Here's how the part is built. I have some questions about the finished solid (model axes, mm). A direction names the side the tool comes from. Coordinates: 2 decimals unless noted, no trailing zeros. Write each loop counter-clockwise with the first axis right and the second up, starting at its lowest first coordinate (ties: lowest second). Pieces come first, ordered by that corner, then holes. Notation, with made-up numbers: (61.5, -33.75) -> (73.5, -33.75) arc R12 cw to (73.5, -27.75) -> close; hole circle Ø4 at (15, 54). An arc over 180 degrees is marked (long way). Answer in a Markdown table with one row per item. Add a question column.
Autodesk Inventor part; units mm, degrees
ref_plane "YZ Plane" through (0, 0, 0) normal (1, 0, 0) x (0, 1, 0)
ref_plane "XZ Plane" through (0, 0, 0) normal (0, 1, 0) x (-1, 0, 0)
ref_plane "XY Plane" through (0, 0, 0) normal (0, 0, 1) x (1, 0, 0)
sketch "Szkic2" plane through (0, 0, 0) normal (0, 1, 0) x (-1, 0, 0)
  line L0 (47.5, 5) -> (-47.5, 5)
  line L1 (-47.5, 5) -> (-47.5, -5)
  line L2 (-47.5, -5) -> (47.5, -5)
  line L3 (47.5, -5) -> (47.5, 5)
  line L4 (47.5, 5) -> (-47.5, -5) construction
  line L5 (-47.5, 5) -> (47.5, -5) construction
  line L6 (0, 24) -> (0, -27)
  point P0 (0, 0)
  dimension "d10" = 10
  dimension "d11" = 95
extrude "Wyciągnięcie proste2" add sketch "Szkic2" along normal blind 1.6
sketch "Szkic3" plane through (0, 1.6, 0) normal (0, 1, 0) x (1, 0, 0)
  line L0 (-47.5, -5) -> (47.5, -5)
  line L1 (47.5, -5) -> (47.5, 5)
  line L2 (47.5, 5) -> (-47.5, 5)
  line L3 (-47.5, 5) -> (-47.5, -5)
  line L4 (52, -8.65) -> (49.4, -5.35) construction
  line L5 (59.75, -18.7) -> (57.1, -15.35) construction
  line L6 (41.3, -1.65) -> (38.65, 1.7) construction
  line L7 (58.425, -17.025) -> (50.7, -7) construction
  line L8 (39.975, 0.025) -> (50.7, -7) construction
  line L9 (58.425, -17.025) -> (58.425, -30) construction
  line L10 (38.5214, -5) -> (47.2545, -10.7203)
  line L11 (47.2545, -10.7203) -> (53.425, -18.728)
  line L12 (53.425, -18.728) -> (53.425, -27.025)
  line L13 (41.5049, 5) -> (54.1455, -3.2797)
  line L14 (54.1455, -3.2797) -> (63.425, -15.322)
  line L15 (63.425, -15.322) -> (63.425, -27.025)
  line L16 (63.425, -27.025) -> (53.425, -27.025)
  line L17 (0, -5) -> (0, 20.232)
  line L18 (-38.5214, -5) -> (-47.2545, -10.7203)
  line L19 (-47.2545, -10.7203) -> (-53.425, -18.728)
  line L20 (-53.425, -18.728) -> (-53.425, -27.025)
  line L21 (-41.5049, 5) -> (-54.1455, -3.2797)
  line L22 (-54.1455, -3.2797) -> (-63.425, -15.322)
  line L23 (-63.425, -15.322) -> (-63.425, -27.025)
  line L24 (-63.425, -27.025) -> (-53.425, -27.025)
  point P0 (0, 0)
  point P1 (-47.5, 1.0732)
  point P2 (47.5, 1.0732)
  dimension "d17" = 5
  dimension "d18" = 5
  dimension "d19" = 10
extrude "Wyciągnięcie proste3" add sketch "Szkic3" against normal up to surface (1.6 mm away) contours L0 L18 L19 L20 L24 L23 L22 L21 L3 | L0 L1 L13 L14 L15 L16 L12 L11 L10
extrude "Wyciągnięcie proste4" cut sketch "Szkic3" against normal through all contours L3 L2 L21 | L2 L1 L13
sketch "Szkic4" plane through (0, 1.6, 0) normal (0, 1, 0) x (1, 0, 0)
  line L0 (-41.5049, 5) -> (-54.1455, -3.2797)
  line L1 (-54.1455, -3.2797) -> (-63.425, -15.322)
  line L2 (-63.425, -15.322) -> (-63.425, -27.025)
  line L3 (-63.425, -27.025) -> (-53.425, -27.025)
  line L4 (-53.425, -27.025) -> (-53.425, -18.728)
  line L5 (-53.425, -18.728) -> (-47.2545, -10.7203)
  line L6 (-47.2545, -10.7203) -> (-38.5214, -5)
  line L7 (-38.5214, -5) -> (38.5214, -5)
  line L8 (38.5214, -5) -> (47.2545, -10.7203)
  line L9 (47.2545, -10.7203) -> (53.425, -18.728)
  line L10 (53.425, -18.728) -> (53.425, -27.025)
  line L11 (53.425, -27.025) -> (63.425, -27.025)
  line L12 (63.425, -27.025) -> (63.425, -15.322)
  line L13 (63.425, -15.322) -> (54.1455, -3.2797)
  line L14 (54.1455, -3.2797) -> (41.5049, 5)
  line L15 (41.5049, 5) -> (-41.5049, 5)
  line L16 (41.5049, 5) -> (35.3982, 9)
  line L17 (35.3982, 9) -> (-35.3982, 9)
  line L18 (-35.3982, 9) -> (-41.5049, 5)
  point P0 (0, 0)
  dimension "d24" = 4
extrude "Wyciągnięcie proste5" add sketch "Szkic4" against normal up to surface (1.6 mm away) contours L18 L17 L16 L15
sketch "Szkic5" plane through (0, 1.6, 0) normal (0, 1, 0) x (1, 0, 0)
  line L0 (-35.3982, 9) -> (-54.1455, -3.2797)
  line L1 (-54.1455, -3.2797) -> (-63.425, -15.322)
  line L2 (-63.425, -15.322) -> (-63.425, -27.025)
  line L3 (-63.425, -27.025) -> (-53.425, -27.025)
  line L4 (-53.425, -27.025) -> (-53.425, -18.728)
  line L5 (-53.425, -18.728) -> (-47.2545, -10.7203)
  line L6 (-47.2545, -10.7203) -> (-38.5214, -5)
  line L7 (-38.5214, -5) -> (38.5214, -5)
  line L8 (38.5214, -5) -> (47.2545, -10.7203)
  line L9 (47.2545, -10.7203) -> (53.425, -18.728)
  line L10 (53.425, -18.728) -> (53.425, -27.025)
  line L11 (53.425, -27.025) -> (63.425, -27.025)
  line L12 (63.425, -27.025) -> (63.425, -15.322)
  line L13 (63.425, -15.322) -> (54.1455, -3.2797)
  line L14 (54.1455, -3.2797) -> (35.3982, 9)
  line L15 (35.3982, 9) -> (-35.3982, 9)
  line L16 (-17, -5) -> (17, -5)
  line L17 (17, -5) -> (17, -15)
  line L18 (17, -15) -> (-17, -15)
  line L19 (-17, -15) -> (-17, -5)
  point P0 (0, 0)
  point P1 (0, -5)
  point P2 (0, 0)
  point P3 (0, -5)
  point P4 (0, -5)
  dimension "d27" = 34
  dimension "d28" = 10
extrude "Wyciągnięcie proste6" add sketch "Szkic5" against normal up to surface (1.6 mm away) contours L7 L17 L18 L19
fillet "Zaokrąglenie1" radius 10 12 edges at (-63.425, 0.8, 15.322) (-54.1455, 0.8, 3.2797) (-35.3982, 0.8, -9) (35.3982, 0.8, -9) (54.1455, 0.8, 3.2797) (63.425, 0.8, 15.322) (-53.425, 0.8, 18.728) (-47.2545, 0.8, 10.7203) (-38.5214, 0.8, 5) (38.5214, 0.8, 5) (47.2545, 0.8, 10.7203) (53.425, 0.8, 18.728)
fillet "Zaokrąglenie2" radius 4 2 edges at (-17, 0.8, 5) (17, 0.8, 5)
fillet "Zaokrąglenie3" radius 2 2 edges at (17, 0.8, 15) (-17, 0.8, 15)
sketch "Szkic6" plane through (0, 1.6, 0) normal (0, 1, 0) x (1, 0, 0)
  line L0 (32.4146, 9) -> (-32.4146, 9)
  line L1 (-5, 9) -> (5, 9)
  line L2 (5, 9) -> (5, 29)
  line L3 (5, 29) -> (-5, 29)
  line L4 (-5, 29) -> (-5, 9)
  point P0 (0, 0)
  point P1 (0, 9)
  point P2 (0, 9)
  dimension "d34" = 10
  dimension "d35" = 20
extrude "Wyciągnięcie proste7" add sketch "Szkic6" against normal up to surface (1.6 mm away)
fillet "Zaokrąglenie4" radius 4 2 edges at (5, 0.8, -9) (-5, 0.8, -9)
fillet "Zaokrąglenie5" radius 1 2 edges at (5, 0.8, -29) (-5, 0.8, -29)
fillet "Zaokrąglenie6" radius 1 4 edges at (-63.425, 0.8, 27.025) (-53.425, 0.8, 27.025) (53.425, 0.8, 27.025) (63.425, 0.8, 27.025)
sketch "Szkic7" plane through (0, 1.6, 0) normal (0, 1, 0) x (1, 0, 0)
  line L0 (-15, -15) -> (15, -15)
  line L1 (17, -13) -> (17, -9)
  line L2 (-17, -9) -> (-17, -13)
  point P0 (0, 0)
  point P1 (-13, -5)
  point P2 (13, -5)
  dimension "d41" = 10
  dimension "d42" = 10
  dimension "d43" = 4
  dimension "d44" = 4
hole "Otwór1" at (-13, 1.6, 5) at (13, 1.6, 5) direction (0, -1, 0) diameter 3.1 depth 15 tip angle 118
properties part number "przód V2.0"
Q1. Imagine slicing it at C-C on z = -22.5. Please give me the cut outline in (x, y), plus the area to 3 significant figures.
Q2. Imagine slicing it at D-D on x = 44. Please give me the cut outline in (y, z), plus the area to 3 significant figures.
Q3. Imagine slicing it at B-B on y = 0.7. State how many separate pieces and enclosed holes the cut face has, plus the area to 3 significant figures.
Q4. For faces 1 (the flat face through (-49.794, 0.811, 14.016)), 2 (the cylindrical face through (6.203, 0.789, -10.141)), which set-ups out of +Z, -Z, +X, -X, +Y, -Y let a thin tool reach every point of the face, with its end or its side?
Q5. If we mould it in two halves opening along Z, with no side actions, what happens to faces 3 (the flat face through (49.794, 0.811, 14.016)), 4 (the flat face through (-1, 0, 5)), 5 (the cylindrical face through (12.93, 0.79, 3.45))? For each: pulls with the +Z half, pulls with the -Z half, needs draft (parallel to the pull), parting line crosses it, or undercut.
Q6. I need wall thicknesses on line 1 (Z direction, x = -13, y = 0.95); line 2 (X direction, y = 0.9, z = 12); line 3 (Z direction, x = 10.5, y = 0.55). Which ranges of each line are inside material? Lowest first, please. Write a range as [from, to].
Q7. Imagine slicing it at A-A on x = 13. Please give me the cut outline in (y, z), plus the area to 3 significant figures.
Q8. I'm going to push flat-ended pins straight in: P1, Ø0.5, axis at y = 1, z = 12, coming from the +X side; P2, Ø0.8, axis at x = -2.5, y = 1, coming from the +Z side; P3, Ø0.8, axis at x = 29, y = 1, coming from the +Z side. Where does each tip first touch, or does it pass through?
Result sheet:
| question | item | result |
|---|---|---|
| 1 | outline | (-5, 0) -> (5, 0) -> (5, 1.6) -> (-5, 1.6) -> close |
| 1 | area | 16.0 mm^2 |
| 2 | outline | (0, -3.37) -> (1.6, -3.37) -> (1.6, 8.59) -> (0, 8.59) -> close |
| 2 | area | 19.1 mm^2 |
| 3 | separate pieces | 1 |
| 3 | enclosed holes | 2 |
| 3 | area | 2,350 mm^2 |
| 4 | face 1 | +Z, +Y, -Y |
| 4 | face 2 | -Z, +X, +Y, -Y |
| 5 | face 3 | pulls with the +Z half |
| 5 | face 4 | needs draft |
| 5 | face 5 | undercut |
| 6 | line 1 | z = [-9, 3.45], [6.55, 15] |
| 6 | line 2 | x = [-60.87, -48.24], [-17, 17], [48.24, 60.87] |
| 6 | line 3 | z = [-9, 15] |
| 7 | outline | (0, -9) -> (1.6, -9) -> (1.6, 3.45) -> (0, 3.45) -> close; (0, 6.55) -> (1.6, 6.55) -> (1.6, 15) -> (0, 15) -> close |
| 7 | area | 33.4 mm^2 |
| 8 | P1 | stops at x = 61.06 |
| 8 | P2 | stops at z = 15 |
| 8 | P3 | stops at z = 5 |
